Geometry check sheet. Reference: the model listing, model coordinates, mm. Face numbers are marked on the shaded views. A direction names the side the tool comes from. Round coordinates to 2 decimals unless told otherwise and drop trailing zeros. Write each loop counter-clockwise with the first axis right and the second up, starting at its lowest first coordinate (ties: lowest second). Pieces come first, ordered by that corner, then holes. Notation, with made-up numbers: M 11.5,-21.5 L 32.5,-21.5 A26 cw 32.5,-3.5 Z; hole C 23.5,40.25 d5. An arc over 180 degrees is marked long. Put each result on its own line as item: value. Start each with the question number.
(1) Section check A-A on x = -13.5. Record the cut outline in (y, z), then the cut area to 3 significant figures.
(2) Mould release check, pull along Y, two halves, no side actions. Record for the marked faces 4, 5, 6 and 7: pulls with the +Y half, pulls with the -Y half, needs draft (parallel to the pull), parting line crosses it, or undercut.
(3) Gauge pin test, flat ends, axial feed: pin 1 (0.7 mm diameter, centred on y = 39, z = -11.5, fed in from -X); pin 2 (9.5 mm diameter, centred on x = 3.5, y = 43.5, fed in from +Z); pin 3 (3 mm diameter, centred on x = 30.5, y = 5, fed in from +Z). Record the tip position at first contact, or that the pin passes through.
(4) Material ranges on probe 1 along X at (y, z) = (2, 0); probe 2 along Y at (x, z) = (0, 20); probe 3 along Y at (x, z) = (0, -19.55), recorded low to high.
(5) Tool access check on the marked faces 1, 2 and 3. Record the directions out of +Z, -Z, +X, -X, +Y, -Y that give a thin tool (end or side, any length) a straight path to the whole face; none if there is none.
(6) Section check C-C on z = -9.5. Record the cut outline in (x, y).
(7) Section check B-B on y = 5.08. Count the separate pieces of the cut face and the enclosed holes in it, then the cut area to 3 significant figures.
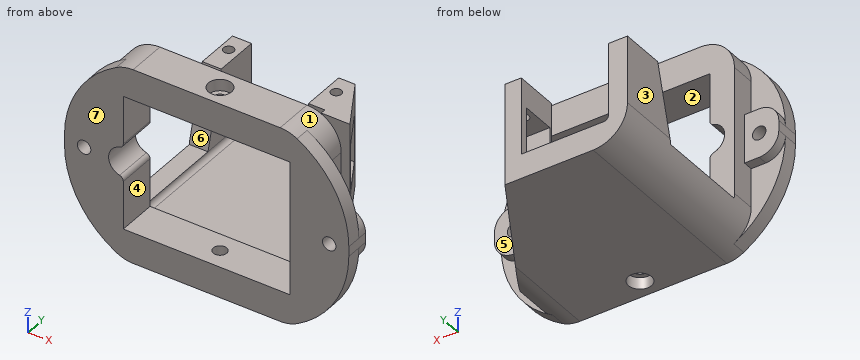
from build123d import *

# Parameters (mm, degrees)
SKETCH1_W           = 55.88
SKETCH1_H           = 50.8
SKETCH1_W_2         = 43.18
SKETCH1_H_2         = 34.798
BOSS_EXTRUDE1_DEPTH = 10.16
SKETCH2_R           = 1.75
CUT_EXTRUDE1_DEPTH  = 59.860081549
SKETCH3_R           = 3
CUT_EXTRUDE2_DEPTH  = 3
SKETCH4_W           = 4.9022
SKETCH4_H           = 20.0152
BOSS_EXTRUDE2_DEPTH = 40.64
CUT_EXTRUDE3_DEPTH  = 77.318648395
FILLET1_R           = 8.89
CHAMFER2_SIZE2      = 40.64
CHAMFER2_SIZE       = 23.46351494
SKETCH6_W           = 4.2418
SKETCH6_H           = 11.487238798
BOSS_EXTRUDE3_DEPTH = 20.0152
BOSS_EXTRUDE5_DEPTH = 20.0152
SKETCH9_R           = 1.35
CUT_EXTRUDE4_DEPTH  = 8
FILLET2_R           = 1.27
BOSS_EXTRUDE6_DEPTH = 6.35
SKETCH11_R          = 1.75
CUT_EXTRUDE5_DEPTH  = 25.4
BOSS_EXTRUDE7_DEPTH = 3.81
CUT_EXTRUDE6_REACH  = 76.62
SKETCH13_W          = 12
SKETCH13_H          = 8.848420696
CUT_EXTRUDE9_REACH  = 62.442
FILLET3_R           = 1.27


# Some blends are built 0.0001 mm under size
with BuildPart() as part:
    # Sketch1 → Boss-Extrude1 (new body)
    with BuildSketch(Plane(origin=(0, 0, 0), x_dir=(1, 0, 0), z_dir=(0, 1, 0))):
        Rectangle(SKETCH1_W, SKETCH1_H)
        Rectangle(SKETCH1_W_2, SKETCH1_H_2, mode=Mode.SUBTRACT)
    extrude(amount=BOSS_EXTRUDE1_DEPTH)

    # Sketch2 → Cut-Extrude1 (cut, through all)
    with BuildSketch(Plane.XY.offset(25.4)):
        with Locations((0, 5.08)):
            Circle(SKETCH2_R)
    extrude(amount=-CUT_EXTRUDE1_DEPTH, mode=Mode.SUBTRACT)

    # Sketch3 → Cut-Extrude2 (cut)
    with BuildSketch(Plane.XY.offset(25.4)):
        with Locations((0, 5.08)):
            Circle(SKETCH3_R)
    cut_extrude2 = extrude(amount=-CUT_EXTRUDE2_DEPTH, mode=Mode.SUBTRACT)

    # Sketch4 → Boss-Extrude2 (add)
    with BuildSketch(Plane(origin=(0, 10.16, 0), x_dir=(1, 0, 0), z_dir=(0, 1, 0))):
        with Locations((-25.4889, 9.0424)):
            Rectangle(SKETCH4_W, SKETCH4_H)
        Polygon((3.81, 25.4), (-27.94, 25.4), (-27.94, 19.05), (-23.0378, 19.05), (3.81, 19.05), align=None)
    extrude(amount=BOSS_EXTRUDE2_DEPTH)

    # Sketch5 → Cut-Extrude3 (cut, through all)
    with BuildSketch(Plane(origin=(-23.0378, 0, 0), x_dir=(0, 0, -1), z_dir=(1, 0, 0))):
        Polygon((17.78, 34.29), (-0.9652, 39.312761202), (-0.9652, 10.16), (17.78, 10.16), align=None)
    extrude(amount=-CUT_EXTRUDE3_DEPTH, mode=Mode.SUBTRACT)

    # Fillet1
    # the kernel refuses this fillet: 8.89 mm, written as the material it takes off along each edge
    with BuildSketch(Plane(origin=(-27.94, -22.225, 25.4), x_dir=(1, 0, 0), z_dir=(0, 1, 0)), Plane(origin=(27.94, -22.225, -25.4), x_dir=(-1, 0, 0), z_dir=(0, 1, 0))) as fillet1_piece_1:
        with BuildLine():
            CenterArc((FILLET1_R, FILLET1_R), FILLET1_R, 180, 90)
            Line((0, FILLET1_R), (0, 0))
            Line((0, 0), (FILLET1_R, 0))
        make_face()
    extrude(amount=54.61, mode=Mode.SUBTRACT)
    with BuildSketch(Plane(origin=(-27.94, -22.225, -25.4), x_dir=(1, 0, 0), z_dir=(0, 1, 0))) as fillet1_piece_2:
        with BuildLine():
            CenterArc((FILLET1_R, -FILLET1_R), FILLET1_R, 90, 90)
            Line((0, -FILLET1_R), (0, 0))
            Line((0, 0), (FILLET1_R, 0))
        make_face()
    extrude(amount=95.25, mode=Mode.SUBTRACT)
    with BuildSketch(Plane(origin=(27.94, -22.225, 25.4), x_dir=(-1, 0, 0), z_dir=(0, 1, 0))) as fillet1_piece_3:
        with BuildLine():
            CenterArc((FILLET1_R, -FILLET1_R), FILLET1_R, 90, 90)
            Line((0, -FILLET1_R), (0, 0))
            Line((0, 0), (FILLET1_R, 0))
        make_face()
    extrude(amount=54.61, mode=Mode.SUBTRACT)

    # Chamfer2
    chamfer2_edges = [part.edges().sort_by_distance(p)[0] for p in [
        (3.81, 10.16, -22.225),
    ]]
    chamfer2_side = [part.faces().sort_by_distance(p)[0] for p in [
        (4.279270299, 10.16, -22.225),
    ]]
    chamfer(chamfer2_edges, length=CHAMFER2_SIZE - 0.0001, length2=CHAMFER2_SIZE2 - 0.0001, reference=chamfer2_side[0])  # a hair under: the kernel refuses the full size

    # Sketch6 → Boss-Extrude3 (add)
    with BuildSketch(Plane.XY.offset(-19.05)):
        with Locations((1.6891, 45.056380601)):
            Rectangle(SKETCH6_W, SKETCH6_H)
    extrude(amount=BOSS_EXTRUDE3_DEPTH)

    # Sketch8 → Boss-Extrude5 (add)
    with BuildSketch(Plane.XY.offset(-19.05)):
        Polygon((3.81, 50.8), (3.81, 37.951579304), (11.228039147, 37.951579304), align=None)
    extrude(amount=BOSS_EXTRUDE5_DEPTH)

    # Sketch9 → Cut-Extrude4 (cut)
    with BuildSketch(Plane.XY.offset(0.9652)):
        with Locations((2.13195, 46.132)):
            Circle(SKETCH9_R)
        with Locations((-25.76195, 46.132)):
            Circle(SKETCH9_R)
    extrude(amount=-CUT_EXTRUDE4_DEPTH, mode=Mode.SUBTRACT)

    # Fillet2
    fillet2_edges = [part.edges().sort_by_distance(p)[0] for p in [
        (-23.0378, 30.48, -19.05),
    ]]
    fillet(fillet2_edges, radius=FILLET2_R)

    # Mirror1: Cut-Extrude2 across plane
    add(cut_extrude2.mirror(Plane.XY), mode=Mode.SUBTRACT)

    # Sketch10 → Boss-Extrude6 (add)
    with BuildSketch(Plane.XZ):
        with BuildLine():
            Line((-27.94, 0), (-27.94, 6.35))
            Line((-27.94, 6.35), (-31.75, 6.35))
            ThreePointArc((-31.75, 6.35), (-35.342102448, 4.862102448), (-36.83, 1.27))
            Line((-36.83, 1.27), (-36.83, -1.27))
            ThreePointArc((-36.83, -1.27), (-35.342102448, -4.862102448), (-31.75, -6.35))
            Line((-31.75, -6.35), (-27.94, -6.35))
            Line((-27.94, -6.35), (-27.94, 0))
        make_face()
    boss_extrude6 = extrude(amount=-BOSS_EXTRUDE6_DEPTH)

    # Mirror2: Boss-Extrude6 across plane
    add(boss_extrude6.mirror(Plane(origin=(0, 0, 0), x_dir=(0, 0, 1), z_dir=(1, 0, 0))))

    # Sketch11 → Cut-Extrude5 (cut)
    with BuildSketch(Plane.XZ):
        with Locations(Location((-31.75, 0, 0), (0, 0, 270))):
            Circle(SKETCH11_R)
        with Locations(Location((31.75, 0, 0), (0, 0, 270))):
            Circle(SKETCH11_R)
    extrude(amount=-CUT_EXTRUDE5_DEPTH, mode=Mode.SUBTRACT)

    # Sketch12 → Boss-Extrude7 (add)
    with BuildSketch(Plane.XZ):
        with BuildLine():
            ThreePointArc((-27.94, 16.51), (-26.728994429, 20.989413417), (-23.425906736, 24.248445596))
            ThreePointArc((-23.425906736, 24.248445596), (-33.234054886, 14.57111535), (-36.83, 1.27))
            ThreePointArc((-36.83, 1.27), (-35.342102448, 4.862102448), (-31.75, 6.35))
            Line((-31.75, 6.35), (-27.94, 6.35))
            Line((-27.94, 6.35), (-27.94, 16.51))
        make_face()
        with BuildLine():
            ThreePointArc((-31.75, -6.35), (-35.342102448, -4.862102448), (-36.83, -1.27))
            ThreePointArc((-36.83, -1.27), (-33.234054886, -14.57111535), (-23.425906736, -24.248445596))
            ThreePointArc((-23.425906736, -24.248445596), (-26.728994429, -20.989413417), (-27.94, -16.51))
            Line((-27.94, -16.51), (-27.94, -6.35))
            Line((-27.94, -6.35), (-31.75, -6.35))
        make_face()
        with BuildLine():
            ThreePointArc((23.425906736, -24.248445596), (33.234054886, -14.57111535), (36.83, -1.27))
            ThreePointArc((36.83, -1.27), (35.342102448, -4.862102448), (31.75, -6.35))
            Line((31.75, -6.35), (27.94, -6.35))
            Line((27.94, -6.35), (27.94, -16.51))
            ThreePointArc((27.94, -16.51), (26.728994429, -20.989413417), (23.425906736, -24.248445596))
        make_face()
        with BuildLine():
            ThreePointArc((36.83, 1.27), (33.234054886, 14.57111535), (23.425906736, 24.248445596))
            ThreePointArc((23.425906736, 24.248445596), (26.728994429, 20.989413417), (27.94, 16.51))
            Line((27.94, 16.51), (27.94, 6.35))
            Line((27.94, 6.35), (31.75, 6.35))
            ThreePointArc((31.75, 6.35), (35.342102448, 4.862102448), (36.83, 1.27))
        make_face()
    extrude(amount=-BOSS_EXTRUDE7_DEPTH)

    # Sketch13 → Cut-Extrude6 (cut, up to next)
    with BuildSketch(Plane.ZY.offset(-11.5682), mode=Mode.PRIVATE) as cut_extrude6_sk1:
        with Locations((-11.7348, 44.375789652)):
            Rectangle(SKETCH13_W, SKETCH13_H)
    cut_extrude6_tool1 = extrude(cut_extrude6_sk1.sketch, amount=CUT_EXTRUDE6_REACH, mode=Mode.PRIVATE) & part.part
    add(cut_extrude6_tool1.solids().sort_by_distance((11.5682, 44.37579, -11.7348))[0], mode=Mode.SUBTRACT)

    # Sketch15 → Cut-Extrude9 (cut, up to next)
    with BuildSketch(Plane(origin=(0, 10.16, 0), x_dir=(1, 0, 0), z_dir=(0, 1, 0)), mode=Mode.PRIVATE) as cut_extrude9_sk1:
        with BuildLine():
            Line((-21.59, 3.81), (-21.59, -3.81))
            ThreePointArc((-21.59, -3.81), (-25.4, 0), (-21.59, 3.81))
        make_face()
    cut_extrude9_tool1 = extrude(cut_extrude9_sk1.sketch, amount=-CUT_EXTRUDE9_REACH, mode=Mode.PRIVATE) & part.part
    add(cut_extrude9_tool1.solids().sort_by_distance((-23.207014, 10.16, 0))[0], mode=Mode.SUBTRACT)

    # Fillet3
    fillet3_edges = [part.edges().sort_by_distance(p)[0] for p in [
        (-21.59, 5.08, 3.81),
        (-21.59, 5.08, -3.81),
    ]]
    fillet(fillet3_edges, radius=FILLET3_R)


solid = part.part
Answers follow:
1. outline: M 0,-25.4 L 50.8,-25.4 L 50.8,-19.05 L 10.16,-19.05 L 10.16,-17.4 L 0,-17.4 Z; M 0,17.4 L 10.16,17.4 L 10.16,25.4 L 0,25.4 Z
1. area: 421 mm^2
2. face 4: needs draft
2. face 5: pulls with the +Y half
2. face 6: undercut
2. face 7: pulls with the -Y half
3. pin 1: stops at x = -27.94
3. pin 2: stops at z = 0.97
3. pin 3: stops at z = 19.43
4. probe 1: x = -36.83 to -33.5, -30 to -25.4, 21.59 to 30, 33.5 to 36.83
4. probe 2: y = 0 to 3.33, 6.83 to 10.16
4. probe 3: y = 0 to 3.33, 6.83 to 50.8
5. face 1: +Z, +X, +Y
5. face 2: +Y, -Y
5. face 3: +Z, -Z, -X, +Y
6. outline: M -35.51,0 L -21.59,0 L -21.59,10.16 L -27.94,10.16 L -27.94,3.81 L -35.51,3.81 Z; M -27.94,36.51 L -23.04,36.51 L -23.04,50.8 L -27.94,50.8 Z; M -0.43,39.31 L 3.81,39.31 L 3.81,37.95 L 11.23,37.95 L 10.07,39.95 L -0.43,39.95 Z; M -0.43,48.8 L 4.96,48.8 L 3.81,50.8 L -0.43,50.8 Z; M 21.59,0 L 35.51,0 L 35.51,3.81 L 27.94,3.81 L 27.94,10.16 L 21.59,10.16 Z
7. separate pieces: 2
7. enclosed holes: 2
7. area: 1,360 mm^2
